from build123d import *

# Parameters (mm, degrees)
SKETCH001_W     = 106
SKETCH001_H     = 54
PAD_DEPTH       = 5
SKETCH_W        = 102
SKETCH_H        = 50
POCKET_DEPTH    = 3
SKETCH002_R     = 2
POCKET001_DEPTH = 2
SKETCH004_W     = 14
SKETCH004_H     = 3
POCKET002_DEPTH = 5
SKETCH005_W     = 2
SKETCH005_H     = 54
PAD001_DEPTH    = 14
SKETCH006_W     = 48
SKETCH006_H     = 13
POCKET003_DEPTH = 2
SKETCH007_W     = 102
SKETCH007_H     = 2
PAD002_DEPTH    = 14
SKETCH008_W     = 102
SKETCH008_H     = 2
PAD003_DEPTH    = 14


with BuildPart() as part:
    # Sketch001 → Pad (new body)
    with BuildSketch(Plane.XY):
        Rectangle(SKETCH001_W, SKETCH001_H)
    extrude(amount=-PAD_DEPTH)

    # Sketch → Pocket (cut)
    with BuildSketch(Plane.XY):
        Rectangle(SKETCH_W, SKETCH_H)
    extrude(amount=-POCKET_DEPTH, mode=Mode.SUBTRACT)

    # Sketch002 (on Face3 of Pocket) → Pocket001 (cut)
    with BuildSketch(Plane.YZ.offset(53)):
        with Locations((-21, 0)):
            Circle(SKETCH002_R)
    extrude(amount=-POCKET001_DEPTH, mode=Mode.SUBTRACT)

    # Sketch004 (on Face6 of Pocket) → Pocket002 (cut)
    with BuildSketch(Plane.XZ.offset(27)):
        with Locations((-31, 0.5)):
            Rectangle(SKETCH004_W, SKETCH004_H)
    extrude(amount=-POCKET002_DEPTH, mode=Mode.SUBTRACT)

    # Sketch005 (on Face4 of Pocket002) → Pad001 (join)
    with BuildSketch(Plane.XY):
        with Locations((-52, 0)):
            Rectangle(SKETCH005_W, SKETCH005_H)
    extrude(amount=PAD001_DEPTH)

    # Sketch006 (on Face8 of Pad001) → Pocket003 (cut)
    with BuildSketch(Plane(origin=(-53, 0, 0), x_dir=(0, -1, 0), z_dir=(-1, 0, 0))):
        with Locations((0, 7.5)):
            Rectangle(SKETCH006_W, SKETCH006_H)
    extrude(amount=-POCKET003_DEPTH, mode=Mode.SUBTRACT)

    # Sketch007 (on Face5 of Pocket003) → Pad002 (join)
    with BuildSketch(Plane.XY):
        with Locations((0, 26)):
            Rectangle(SKETCH007_W, SKETCH007_H)
    extrude(amount=PAD002_DEPTH)

    # Sketch008 (on Face11 of Pad002) → Pad003 (join)
    with BuildSketch(Plane.XY):
        with Locations((0, -26)):
            Rectangle(SKETCH008_W, SKETCH008_H)
    extrude(amount=PAD003_DEPTH)


solid = part.part
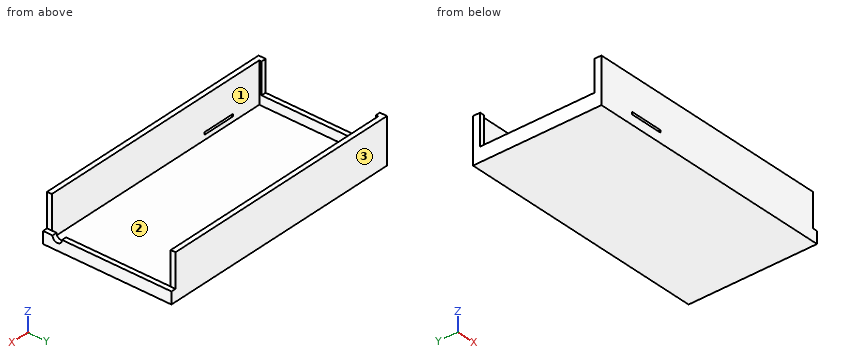
Design review of the part built by this model. Coordinates are the model's own, in mm. Face numbers are marked on the shaded views. Coordinates: 2 decimals unless noted, no trailing zeros. Write each loop counter-clockwise with the first axis right and the second up, starting at its lowest first coordinate (ties: lowest second). Pieces come first, ordered by that corner, then holes. Notation, with made-up numbers: (-19.5, -13.5) - (-4.5, -13.5) arc R16 cw to (-4.5, -3.5) - close; hole circle Ø11 at (23.25, 52). An arc over 180 degrees is marked (long way). Use one line per item in the form item = value.
Q1. The part is to be moulded in two halves that separate along X. For the marked faces 1, 2 and 3, say which applies: +X half, -X half, draft (parallel to the pull), parting line (faces both ways), or undercut.
Taken from the geometry:
face_1 = undercut
face_2 = undercut
face_3 = draft
Q2. For probe 1 along Y at (x, z) = (-29, 0.5); probe 2 along X at (y, z) = (23, -1); probe 3 along Z at (x, y) = (-32.5, 22.5), list the stretches that pass through material, from the lowest coordinate up.
Taken from the geometry:
probe_1 = -27 to -25, 25 to 27
probe_2 = -53 to -51, 51 to 53
probe_3 = -5 to -3
Q3. Consider section B-B (y = 14). Write out the cut boundary in (x, z), plus the area to 3 significant figures.
Taken from the geometry:
outline = (-53, -5) - (53, -5) - (53, 0) - (51, 0) - (51, -3) - (-51, -3) - (-51, 1) - (-53, 1) - close
area = 226 mm^2
Q4. Consider section C-C (x = -8). Write out the cut boundary in (y, z), plus the area to 3 significant figures.
Taken from the geometry:
outline = (-27, -5) - (27, -5) - (27, 14) - (25, 14) - (25, -3) - (-25, -3) - (-25, 14) - (-27, 14) - close
area = 176 mm^2
Q5. Consider section A-A (x = -26). Write out the cut boundary in (y, z), plus the area to 3 significant figures.
Taken from the geometry:
outline = (-27, -5) - (27, -5) - (27, 14) - (25, 14) - (25, -3) - (-25, -3) - (-25, -1) - (-27, -1) - close; (-27, 0) - (-25, 0) - (-25, 14) - (-27, 14) - close
area = 174 mm^2
Q6. Insertion check: pin 1 Ø2 at (x, y) = (51.5, 15.5) entering from +Z; pin 2 Ø1 at (x, y) = (-36.5, -20) entering from +Z; pin 3 Ø2 at (y, z) = (-26, 5.5) entering from +X. Each pin has a flat end and moves straight along its axis. Give the tip position at first contact, or say it passes through.
Taken from the geometry:
pin_1 = 0
pin_2 = -3
pin_3 = 51
